Source: CAD feature listing. Evaluate the final solid. Frame: model axes, mm. Give positions to 0.01 mm unless a question says otherwise; leave off trailing zeros. Order: outer loops, then holes, each group sorted by start corner. A loop starts at its lowest first (then second) coordinate and runs counter-clockwise, first axis right, second up. Notation, with made-up numbers: (-17, 2) - (10, 2) arc R32 cw to (10, 30) - close; hole circle Ø1 at (39, 73). An arc over 180 degrees is marked (long way). Answer as CSV lines item,"result".
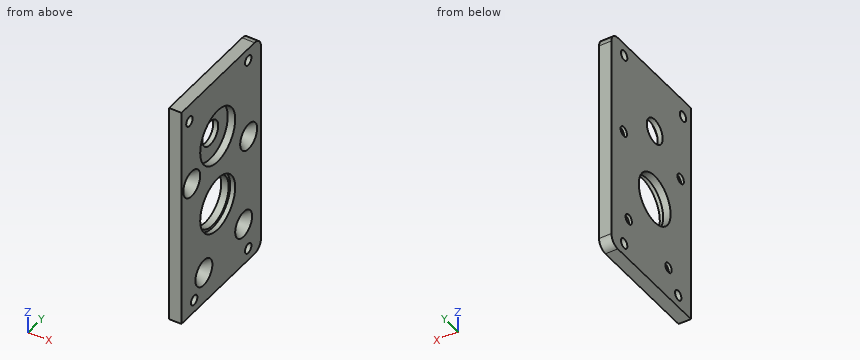
Autodesk Inventor part; units mm, degrees
ref_plane "YZ Plane" through (0, 0, 0) normal (1, 0, 0) x (0, 1, 0)
ref_plane "XZ Plane" through (0, 0, 0) normal (0, 1, 0) x (-1, 0, 0)
ref_plane "XY Plane" through (0, 0, 0) normal (0, 0, 1) x (1, 0, 0)
sketch "Sketch1" plane through (0, 0, 0) normal (1, 0, 0) x (0, 1, 0)
  line L0 (0, 0) -> (50, 0)
  line L1 (50, 0) -> (50, -91)
  line L2 (50, -91) -> (0, -91)
  line L3 (0, -91) -> (0, 0)
  dimension "d0" = 50
  dimension "d1" = 91
extrude "Extrusion1" add sketch "Sketch1" along normal blind 5
sketch "Sketch2" plane through (5, 0, 0) normal (1, 0, 0) x (0, 0, -1)
  line L0 (0, 0) -> (91, 0)
  line L1 (0, 50) -> (0, 0)
  point P0 (25, 22.8)
  dimension "d4" = 22.8
  dimension "d5" = 25
hole "Hole1" at (5, 22.8, -25) direction (-1, 0, 0) diameter 10 end through all counterbore diameter 22 counterbore depth 3
sketch "Sketch3" plane through (5, 0, 0) normal (1, 0, 0) x (0, 0, -1)
  circle A0 centre (25, 22.8) radius 11
  line L0 (91, 0) -> (91, 50)
  line L1 (91, 50) -> (0, 50)
  line L2 (0, 50) -> (0, 0)
  line L3 (0, 0) -> (91, 0)
  circle A1 centre (25, 22.8) radius 5
  line L4 (25, 22.8) -> (54.26, 22.8)
  dimension "d13" = 29.26
  dimension "d14" = 0
hole "Hole2" at (5, 22.8, -54.26) direction (-1, 0, 0) diameter 20 end through all counterbore diameter 22 counterbore depth 2
sketch "Sketch4" plane through (5, 0, 0) normal (1, 0, 0) x (0, 0, -1)
  circle A0 centre (54.26, 22.8) radius 11
  line L0 (54.26, 22.8) -> (73.7175, 39.1268)
  line L1 (0, 0) -> (91, 0)
  point P0 (49.8493, 47.8141)
  point P1 (30.3918, 31.4873)
  point P2 (34.8025, 6.4732)
  point P3 (58.6707, -2.2141)
  point P4 (78.1282, 14.1127)
  dimension "d22" = 25.4
  dimension "d23" = 40
  dimension "d33" = 360
hole "Falcon Bolt Holes" at (5, 39.1268, -73.7175) at (5, 6.4732, -34.8025) at (5, 14.1127, -78.1282) direction (-1, 0, 0) diameter 4 end through all countersink diameter 10.668 countersink angle 82
fillet "Fillet1" radius 4 2 edges at (2.5, 50, 0) (2.5, 50, -91)
sketch "Sketch8" plane through (5, 0, 0) normal (1, 0, 0) x (0, 0, -1)
  line L0 (87, 50) -> (4, 50)
  line L1 (91, 0) -> (91, 46)
  line L2 (0, 0) -> (91, 0)
  line L3 (0, 46) -> (0, 0)
  circle A0 centre (5, 42) radius 4.5
  circle A1 centre (5, 42) radius 2
  circle A2 centre (7, 5) radius 4.5
  circle A3 centre (7, 5) radius 2
  circle A4 centre (86, 42) radius 4.5
  circle A5 centre (86, 42) radius 2
  circle A6 centre (86, 8) radius 4.5
  circle A7 centre (86, 8) radius 2
  dimension "d55" = 8
  dimension "d57" = 5
  dimension "d58" = 8
  dimension "d59" = 7
  dimension "d60" = 5
  dimension "d61" = 5
  dimension "d62" = 8
  dimension "d63" = 9
  dimension "d64" = 4
  dimension "d65" = 9
  dimension "d66" = 4
  dimension "d67" = 9
  dimension "d68" = 4
  dimension "d69" = 9
  dimension "d70" = 4
  dimension "d71" = 5
hole "Hole5" at (5, 42, -5) at (5, 42, -86) at (5, 8, -86) at (5, 5, -7) direction (-1, 0, 0) diameter 4 end through all
sketch "Sketch10" plane through (5, 0, 0) normal (1, 0, 0) x (0, 0, -1)
  circle A0 centre (54.26, 22.8) radius 11
  line L0 (37.9332, 42.2575) -> (73.7175, 39.1268)
  line L1 (73.7175, 39.1268) -> (70.5868, 3.3425)
  line L2 (70.5868, 3.3425) -> (34.8025, 6.4732)
  line L3 (34.8025, 6.4732) -> (37.9332, 42.2575)
  line L4 (54.26, 22.8) -> (37.9332, 42.2575)
  line L5 (0, 46) -> (0, 0)
  line L6 (91, 0) -> (91, 46)
  line L7 (0, 0) -> (91, 0)
  circle A1 centre (34.8025, 6.4732) radius 2
  dimension "d81" = 25.4
  dimension "d82" = 5
hole "Neo Bolt Holes" at (5, 42.2575, -37.9332) at (5, 39.1268, -73.7175) at (5, 6.4732, -34.8025) direction (-1, 0, 0) diameter 4 end through all countersink diameter 10.668 countersink angle 82
properties part number "One Motor Plate"
(1) Cut plane C-C (x = 3.9). Give the number of separate pieces and of enclosed holes in the cut face, then the cut area to 3 significant figures.
Completed:
separate pieces,"1"
enclosed holes,"10"
area,"3,490 mm²"
(2) Cut plane B-B (z = -54.26). Return loops of the section in (x, y).
Completed:
outline,"(0, 0) - (5, 0) - (5, 11.8) - (3, 11.8) - (3, 12.8) - (0, 12.8) - close; (0, 32.8) - (3, 32.8) - (3, 33.8) - (5, 33.8) - (5, 50) - (0, 50) - close"
(3) Ray query, line 1 (Z direction, x = 3.7, y = 22.8); line 2 (Z direction, x = 2.2, y = 22.8); line 3 (Y direction, x = 2.4, z = -86). Return the intervals inside material, ascending. Write a range as from..to.
Completed:
line 1,"-91..-65.26, -43.26..-36, -14..0"
line 2,"-91..-64.26, -44.26..-36, -14..0"
line 3,"0..6, 10..40, 44..50"
(4) Cut plane D-D (y = 31). Return loops of the section in (x, z).
Completed:
outline,"(0, -91) - (5, -91) - (5, -61.59) - (3, -61.59) - (3, -59.98) - (0, -59.98) - close; (0, -48.54) - (3, -48.54) - (3, -46.93) - (5, -46.93) - (5, -32.33) - (2, -32.33) - (2, -17.67) - (5, -17.67) - (5, 0) - (0, 0) - close"
(5) Contact query for a flat-ended pin moving along its axis: pin 1 (6.5 mm diameter, centred on y = 21.5, z = -23, fed in from +X). Output: stop coordinate, or through.
Completed:
pin 1,"x = 2"
(6) Cut plane A-A (y = 22.8). Return loops of the section in (x, z).
Completed:
outline,"(0, -91) - (5, -91) - (5, -65.26) - (3, -65.26) - (3, -64.26) - (0, -64.26) - close; (0, -44.26) - (3, -44.26) - (3, -43.26) - (5, -43.26) - (5, -36) - (2, -36) - (2, -30) - (0, -30) - close; (0, -20) - (2, -20) - (2, -14) - (5, -14) - (5, 0) - (0, 0) - close"
